Input: dimensioned drawing with shaded views. Units: mm. Origin: part minimum x, y, z. A direction names the side the tool comes from. Coordinates: 2 decimals unless noted, no trailing zeros. Loops run counter-clockwise (first coordinate to the right, second up) from the corner with the lowest first, then second, coordinate; pieces in that order, holes last. Notation, with made-up numbers: M -3,5 L 8,5 A18 ccw 8,39 Z; hole C 12.25,20 d4. An arc over 180 degrees is marked long. Write item = value, one per line. Start each with the question number.
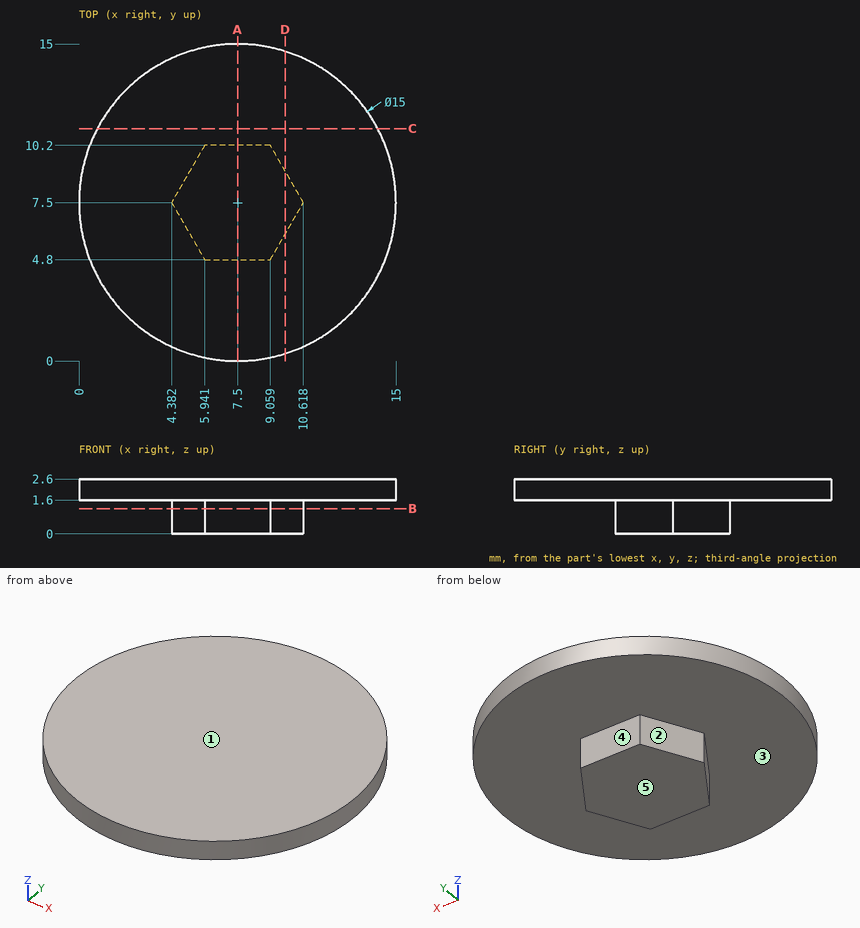
Item 1: Section query D-D (x = 9.75). Return the cut outline in (y, z) (1 decimal), plus the area to 3 significant figures.
Item 2: Line query: line 1 (Y direction, x = 6.5, z = 0.6); line 2 (Z direction, x = 12.25, y = 2); line 3 (X direction, y = 2.5, z = 2.35). Output: solid intervals per line, ascending. Write a range as from..to.
Item 3: First-contact query: pin 1 (1.5 mm diameter, centred on x = 3, z = 1, fed in from +Y). Flat tip, straight axial feed; report the tip coordinate or a pass-through.
Item 4: Reachability of the marked faces 1, 2, 3, 4 and 5 from +Z, -Z, +X, -X, +Y, -Y: full face, straight path, thin tool, end or side. Return the list, or none.
Item 5: Section query A-A (x = 7.5). Return the cut outline in (y, z).
Item 6: Section query B-B (z = 1.2). Return the cut outline in (x, y).
Item 7: Section query C-C (y = 11). Return the cut outline in (x, z).
Verdict:
q1.outline = M 0.3,1.6 L 6,1.6 L 6,0 L 9,0 L 9,1.6 L 14.7,1.6 L 14.7,2.6 L 0.3,2.6 Z
q1.area = 19.1 mm2
q2.line_1 = 4.8..10.2
q2.line_2 = 1.6..2.6
q2.line_3 = 1.91..13.09
q3.pin_1 = 13.81
q4.face_1 = +Z, +X, -X, +Y, -Y
q4.face_2 = -Z, -X, +Y
q4.face_3 = -Z
q4.face_4 = -Z, +X, -X, +Y
q4.face_5 = -Z, +X, -X, +Y, -Y
q5.outline = M 0,1.6 L 4.8,1.6 L 4.8,0 L 10.2,0 L 10.2,1.6 L 15,1.6 L 15,2.6 L 0,2.6 Z
q6.outline = M 4.38,7.5 L 5.94,4.8 L 9.06,4.8 L 10.62,7.5 L 9.06,10.2 L 5.94,10.2 Z
q7.outline = M 0.87,1.6 L 14.13,1.6 L 14.13,2.6 L 0.87,2.6 Z
